from build123d import *

# Parameters (mm, degrees)
SKETCH040_W             = 65
SKETCH040_H             = 30
SKETCH040_R             = 1.45
PAD013_DEPTH            = 1.1
SKETCH042_W             = 14.4
SKETCH042_H             = 17.5
PAD014_DEPTH            = 16
SKETCH043_W             = 16
SKETCH043_H             = 21
PAD015_DEPTH            = 13.8
SKETCH044_W             = 6
SKETCH044_H             = 13.9
PAD016_DEPTH            = 5
SKETCH045_W             = 4.4
SKETCH045_H             = 4.9
SKETCH045_W_2           = 4.5
PAD017_DEPTH            = 4.3
SKETCH046_W             = 6
SKETCH046_H             = 5.4
PAD018_DEPTH            = 8.9
BODY004_PLACEMENT_ANGLE = 180


with BuildPart() as part:
    # Sketch040 → Pad013 (new body)
    with BuildSketch(Plane.XY):
        Rectangle(SKETCH040_W, SKETCH040_H)
        with Locations((-29, 11.5)):
            Circle(SKETCH040_R, mode=Mode.SUBTRACT)
        with Locations((29, 11.5)):
            Circle(SKETCH040_R, mode=Mode.SUBTRACT)
        with Locations((29, -11.5)):
            Circle(SKETCH040_R, mode=Mode.SUBTRACT)
        with Locations((-29, -11.5)):
            Circle(SKETCH040_R, mode=Mode.SUBTRACT)
    extrude(amount=PAD013_DEPTH)

    # Sketch042 (on Face10 of Pad013) → Pad014 (join)
    with BuildSketch(Plane.XY.offset(1.1)):
        with Locations((-17.4, -8.75)):
            Rectangle(SKETCH042_W, SKETCH042_H)
    extrude(amount=PAD014_DEPTH)

    # Sketch043 (on Face5 of Pad014) → Pad015 (join)
    with BuildSketch(Plane.XY.offset(1.1)):
        with Locations((3.3, -7)):
            Rectangle(SKETCH043_W, SKETCH043_H)
    extrude(amount=PAD015_DEPTH)

    # Sketch044 (on Face5 of Pad015) → Pad016 (join)
    with BuildSketch(Plane.XY.offset(1.1)):
        with Locations((21.3, -10.55)):
            Rectangle(SKETCH044_W, SKETCH044_H)
    extrude(amount=PAD016_DEPTH)

    # Sketch045 (on Face5 of Pad016) → Pad017 (join)
    with BuildSketch(Plane.XY.offset(1.1)):
        with Locations((12.6, 14.25)):
            Rectangle(SKETCH045_W, SKETCH045_H)
        with Locations((0.55, 14.25)):
            Rectangle(SKETCH045_W_2, SKETCH045_H)
        with Locations((-11.75, 14.25)):
            Rectangle(SKETCH045_W_2, SKETCH045_H)
    extrude(amount=PAD017_DEPTH)

    # Sketch046 (on Face5 of Pad017) → Pad018 (join)
    with BuildSketch(Plane.XY.offset(1.1)):
        with Locations((-20.9, 13)):
            Rectangle(SKETCH046_W, SKETCH046_H)
    extrude(amount=PAD018_DEPTH)


with BuildPart() as part_1:
    # Body004 placement: moved
    add(part.part.moved(Location((0, 0, 13.5))).rotate(Axis((0, 0, 13.5), (0, 0, 1)), BODY004_PLACEMENT_ANGLE))


solid = part_1.part
Geometry check sheet. Reference: the model listing, model coordinates, mm. A direction names the side the tool comes from. Give positions to 0.01 mm unless a question says otherwise; leave off trailing zeros. Write each loop counter-clockwise with the first axis right and the second up, starting at its lowest first coordinate (ties: lowest second). Pieces come first, ordered by that corner, then holes. Notation, with made-up numbers: M 31,39.25 L 43,39.25 A11 ccw 43,49.25 Z; hole C 57.5,73 d10. An arc over 180 degrees is marked long. Answer as CSV lines item,"result". Start each with the question number.
Q1. Section check D-D, the plane x = 29. Record the cut outline in (y, z).
Q2. Material ranges on L1, parallel to Y at x = -29, z = 14.3; L2, parallel to X at y = 9.5, z = 26; L3, parallel to Z at x = 14, y = -5, recorded low to high.
Q3. Section check B-B, the plane y = 11.5. Record the cut outline in (x, z), then the cut area to 3 significant figures.
Q4. Tool access check on faces 1 (the face through (-2.8, -14, 17)), 2 (the face through (-21, 3.6, 17)), 3 (the face through (10.2, 9, 22)), 4 (the face through (-18.3, 11, 17)), 5 (the face through (12, -11.8, 17)). Record the directions out of +Z, -Z, +X, -X, +Y, -Y that give a thin tool (end or side, any length) a straight path to the whole face; none if there is none.
Q5. Release check for a two-part mould opening along X. For faces 6 (the face through (17.9, -13, 19)), 7 (the face through (12, -14, 18.9)), 8 (the face through (23.9, -13, 19)), 9 (the face through (-14.8, -14, 17)) record: pulls with the +X half, pulls with the -X half, needs draft (parallel to the pull), parting line crosses it, or undercut.
Q6. Section check C-C, the plane z = 20.75. Record the cut outline in (x, y), then the cut area to 3 significant figures.
Q7. Section check A-A, the plane z = 15.5. Record the cut outline in (x, y).
Q8. Go/stop test with flat-tipped pins: pin 1 (1.8 mm diameter, centred on x = 22, z = 21, fed in from -Y); pin 2 (1.7 mm diameter, centred on x = -29, y = -11.5, fed in from +Z); pin 3 (6 mm diameter, centred on y = -2.5, z = 25.5, fed in from -X); pin 4 (1.2 mm diameter, centred on x = -2, y = 16, fed in from -Z). Record where each tip stops, or that it passes through.
Geometry says:
1,outline,"M -15,13.5 L -12.95,13.5 L -12.95,14.6 L -15,14.6 Z; M -10.05,13.5 L 10.05,13.5 L 10.05,14.6 L -10.05,14.6 Z; M 12.95,13.5 L 15,13.5 L 15,14.6 L 12.95,14.6 Z"
2,L1,"-15 to -12.95, -10.05 to 10.05, 12.95 to 15"
2,L2,"-11.3 to 4.7, 10.2 to 24.6"
2,L3,"13.5 to 14.6"
3,outline,"M -32.5,13.5 L -30.45,13.5 L -30.45,14.6 L -32.5,14.6 Z; M -27.55,13.5 L 27.55,13.5 L 27.55,14.6 L 24.6,14.6 L 24.6,30.6 L 10.2,30.6 L 10.2,14.6 L 4.7,14.6 L 4.7,28.4 L -11.3,28.4 L -11.3,14.6 L -18.3,14.6 L -18.3,19.6 L -24.3,19.6 L -24.3,14.6 L -27.55,14.6 Z; M 30.45,13.5 L 32.5,13.5 L 32.5,14.6 L 30.45,14.6 Z"
3,area,"546 mm^2"
4,face 1,"+Z, -Y"
4,face 2,"+Z, -X, -Y"
4,face 3,"+Z, +Y"
4,face 4,"+Z, +Y, -Y"
4,face 5,"+Z, -X"
5,face 6,"undercut"
5,face 7,"needs draft"
5,face 8,"pulls with the +X half"
5,face 9,"pulls with the -X half"
6,outline,"M -11.3,-3.5 L 4.7,-3.5 L 4.7,17.5 L -11.3,17.5 Z; M 10.2,0 L 24.6,0 L 24.6,17.5 L 10.2,17.5 Z; M 17.9,-15.7 L 23.9,-15.7 L 23.9,-10.3 L 17.9,-10.3 Z"
6,area,"620 mm^2"
7,outline,"M -24.3,3.6 L -18.3,3.6 L -18.3,17.5 L -24.3,17.5 Z; M -14.8,-16.7 L -10.4,-16.7 L -10.4,-11.8 L -14.8,-11.8 Z; M -11.3,-3.5 L 4.7,-3.5 L 4.7,17.5 L -11.3,17.5 Z; M -2.8,-16.7 L 1.7,-16.7 L 1.7,-11.8 L -2.8,-11.8 Z; M 9.5,-16.7 L 14,-16.7 L 14,-11.8 L 9.5,-11.8 Z; M 10.2,0 L 24.6,0 L 24.6,17.5 L 10.2,17.5 Z; M 17.9,-15.7 L 23.9,-15.7 L 23.9,-10.3 L 17.9,-10.3 Z"
8,pin 1,"y = -15.7"
8,pin 2,"through"
8,pin 3,"x = -11.3"
8,pin 4,"z = 14.6"
